from build123d import *

# Parameters (mm, degrees)
SALIENTE_EXTRUIR1_DEPTH = 0.1


with BuildPart() as part:
    # Model → Saliente-Extruir1 (new body)
    with BuildSketch(Plane.XY):
        with BuildLine():
            Line((18.549433899, 16.929238501), (35.049433899, 16.929238501))
            Line((35.049433899, 16.929238501), (50.549433899, 16.929238501))
            Line((50.549433899, 16.929238501), (50.549433899, 9.564394878))
            ThreePointArc((50.549433899, 9.564394878), (52.846061309, 11.155038033), (54.613628105, 13.318449858))
            ThreePointArc((54.613628105, 13.318449858), (55.63441871, 15.607287158), (56.05464892, 18.077954318))
            Line((56.05464892, 18.077954318), (47.725070346, 21.375387298))
            Line((47.725070346, 21.375387298), (34.549148093, 17.736158759))
            Line((34.549148093, 17.736158759), (21.373432242, 21.375830254))
            Line((21.373432242, 21.375830254), (13.040093285, 18.077232707))
            ThreePointArc((13.040093285, 18.077232707), (13.464781987, 15.585792102), (14.494191445, 13.277556205))
            ThreePointArc((14.494191445, 13.277556205), (16.258659897, 11.134658879), (18.546640013, 9.562874906))
            Line((18.546640013, 9.562874906), (18.549433899, 16.929238501))
        make_face()
    extrude(amount=SALIENTE_EXTRUIR1_DEPTH)


solid = part.part
Can you work these out from the model? Positions are in its coordinate system, mm. Give positions to 0.01 mm unless a question says otherwise; leave off trailing zeros. Loops run counter-clockwise (first coordinate to the right, second up) from the corner with the lowest first, then second, coordinate; pieces in that order, holes last. Notation, with made-up numbers: (32, -26.5) - (62, -26.5) arc R12 cw to (62, -18.5) - close; hole circle Ø9 at (-39, 58.25). An arc over 180 degrees is marked (long way). One line per item, written item: value.
(1) If we section it at A-A, the plane y = 19.5: List the corners of the cut face in (x, z) for me, plus the area to 3 significant figures.
Verdict:
outline: (16.63, 0) - (28.16, 0) - (28.16, 0.1) - (16.63, 0.1) - close; (40.94, 0) - (52.46, 0) - (52.46, 0.1) - (40.94, 0.1) - close
area: 2.31 mm^2
(2) If we section it at B-B, the plane z = 0.05: List the corners of the cut face in (x, y) for me.
Verdict:
outline: (13.04, 18.08) arc R10.11 ccw to (14.49, 13.28) arc R9.95 ccw to (18.55, 9.56) - (18.55, 16.93) - (50.55, 16.93) - (50.55, 9.56) arc R10.01 ccw to (56.05, 18.08) - (47.73, 21.38) - (34.55, 17.74) - (21.37, 21.38) - close
(3) If we section it at C-C, the plane y = 16.5: List the corners of the cut face in (x, z) for me, plus the area to 3 significant figures.
Verdict:
outline: (13.23, 0) - (18.55, 0) - (18.55, 0.1) - (13.23, 0.1) - close; (50.55, 0) - (55.86, 0) - (55.86, 0.1) - (50.55, 0.1) - close
area: 1.06 mm^2
(4) I need wall thicknesses on line 1 along Y through (x, z) = (52.5, 0.05); line 2 along Y through (x, z) = (26.5, 0.05). Which ranges of each line are inside material? Lowest first, please.
Verdict:
line 1: 10.85 to 19.49
line 2: 16.93 to 19.96
(5) If we section it at D-D, the plane x = 20: List the corners of the cut face in (y, z) for me, plus the area to 3 significant figures.
Verdict:
outline: (16.93, 0) - (20.83, 0) - (20.83, 0.1) - (16.93, 0.1) - close
area: 0.390 mm^2
